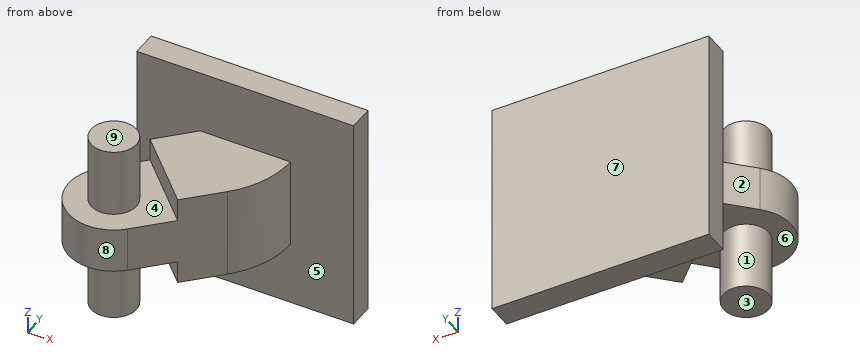
```python
from build123d import *

# Parameters (mm, degrees)
SKETCH_1_W           = 60
SKETCH_1_H           = 60
EXTRUDE_1_DEPTH      = 7
EXTRUDE_2_DEPTH      = 12.5
EXTRUDE_2_DEPTH_BACK = 12.5
CUT_EXTRUDE_START    = -12.5
CUT_EXTRUDE_1_DEPTH  = 6.25
CUT_EXTRUDE_START_2  = 6.25
CUT_EXTRUDE_2_DEPTH  = 6.25
EXTRUDE_3_DEPTH      = 25
EXTRUDE_3_DEPTH_BACK = 25
SKETCH_5_R           = 6.25


with BuildPart() as part:
    # 草图1 → 凸台-拉伸1 (new body)
    with BuildSketch(Plane(origin=(0, 0, 0), x_dir=(1, 0, 0), z_dir=(0, 1, 0))):
        Rectangle(SKETCH_1_W, SKETCH_1_H)
    extrude(amount=EXTRUDE_1_DEPTH)

    # 草图2 → 凸台-拉伸2 (add, two sides: drawn at the far end of the back side and taken through both)
    with BuildSketch(Plane.XY.offset(-EXTRUDE_2_DEPTH_BACK)):
        with BuildLine():
            Line((-12.5, 0), (12.5, 0))
            ThreePointArc((12.5, 0), (10.596988313, -9.567085809), (5.17766953, -17.67766953))
            Line((5.17766953, -17.67766953), (-12.5, -35.355339059))
            ThreePointArc((-12.5, -35.355339059), (-30.17766953, -35.355339059), (-30.17766953, -17.67766953))
            Line((-30.17766953, -17.67766953), (-12.5, 0))
        make_face()
    extrude(amount=EXTRUDE_2_DEPTH + EXTRUDE_2_DEPTH_BACK)

    # 草图3 → 切除-拉伸1 (cut)
    with BuildSketch(Plane.XY.offset(CUT_EXTRUDE_START)):
        with BuildLine():
            Line((-21.338834765, -8.838834765), (-3.661165235, -26.516504294))
            Line((-3.661165235, -26.516504294), (-12.5, -35.355339059))
            ThreePointArc((-12.5, -35.355339059), (-30.17766953, -35.355339059), (-30.17766953, -17.67766953))
            Line((-30.17766953, -17.67766953), (-21.338834765, -8.838834765))
        make_face()
    extrude(amount=CUT_EXTRUDE_1_DEPTH, mode=Mode.SUBTRACT)

    # 草图4 → 切除-拉伸2 (cut)
    with BuildSketch(Plane.XY.offset(CUT_EXTRUDE_START_2)):
        with BuildLine():
            Line((-3.661165235, -26.516504294), (-21.338834765, -8.838834765))
            Line((-21.338834765, -8.838834765), (-30.17766953, -17.67766953))
            ThreePointArc((-30.17766953, -17.67766953), (-30.17766953, -35.355339059), (-12.5, -35.355339059))
            Line((-12.5, -35.355339059), (-3.661165235, -26.516504294))
        make_face()
    extrude(amount=CUT_EXTRUDE_2_DEPTH, mode=Mode.SUBTRACT)

    # 草图5 → 凸台-拉伸3 (add, two sides: drawn at the far end of the back side and taken through both)
    with BuildSketch(Plane.XY.offset(-EXTRUDE_3_DEPTH_BACK)):
        with Locations((-21.338834765, -26.516504294)):
            Circle(SKETCH_5_R)
    extrude(amount=EXTRUDE_3_DEPTH + EXTRUDE_3_DEPTH_BACK)


solid = part.part
```
CAD build for the part. Positions are in the model's coordinates, mm. Face numbers are marked on the shaded views. A direction names the side the tool comes from. Coordinates: 2 decimals unless noted, no trailing zeros. Write each loop counter-clockwise with the first axis right and the second up, starting at its lowest first coordinate (ties: lowest second). Pieces come first, ordered by that corner, then holes. Notation, with made-up numbers: (66.25, 49.25) -> (125.25, 49.25) arc R28 cw to (125.25, 68.25) -> close; hole circle Ø3 at (-0.75, 78). An arc over 180 degrees is marked (long way). Return JSON: item names as keys, results as strings. Group by question number.
Q1. Which spindle directions (+Z, -Z, +X, -X, +Y, -Y) get a long thin tool onto all of the face, cutting with end or side? Do the marked faces 1, 2, 3, 4 and 5. Say none if no direction does.
Q2. Cut at D-D, the plane y = -23.5. Give the cut face in (x, z), then the cut area to 3 significant figures.
Q3. Cut at C-C, the plane z = 4. Give the cut face in (x, y), then the cut area to 3 significant figures.
Q4. Cut at B-B, the plane x = -19. Give the cut face in (y, z).
Q5. Pull direction Y, two halves, no side cores. Call the marked faces 6, 7, 8 and 9: released by +Y, released by -Y, zero draft, split by the parting line, or undercut.
Q6. Drill centre lines: line 1 (Y direction, x = 13.5, z = -9.5); line 2 (Z direction, x = -16.5, y = -35); line 3 (X direction, y = -26.5, z = -15). Where is each one in solid material? Low to high.
Q7. Flat gauge pins, fed straight in: pin 1 (5 mm diameter, centred on y = -8.5, z = 7.5, fed in from -X); pin 2 (13.5 mm diameter, centred on x = -9, y = -18.5, fed in from -Z); pin 3 (2 mm diameter, centred on y = 5, z = 5, fed in from -X). Where does each tip first touch, or does it go through?
Q8. Cut at A-A, the plane z = -10. Give the cut face in (x, y).
Returned:
{
 "1": {"face 1": "-Z", "face 2": "+Z, -Z, -X", "face 3": "-Z, +X, -X, -Y", "face 4": "+Z", "face 5": "none"},
 "2": {"outline": "(-33.47, -6.25) -> (-26.81, -6.25) -> (-26.81, -25) -> (-15.86, -25) -> (-15.86, -6.25) -> (-6.68, -6.25) -> (-6.68, -12.5) -> (-0.64, -12.5) -> (-0.64, 12.5) -> (-6.68, 12.5) -> (-6.68, 6.25) -> (-15.86, 6.25) -> (-15.86, 25) -> (-26.81, 25) -> (-26.81, 6.25) -> (-33.47, 6.25) -> close", "area": "896 mm2"},
 "3": {"outline": "(-30.18, -17.68) arc R12.5 ccw to (-12.5, -35.36) -> (5.18, -17.68) arc R25 ccw to (12.5, 0) -> (30, 0) -> (30, 7) -> (-30, 7) -> (-30, 0) -> (-12.5, 0) -> close", "area": "1,540 mm2"},
 "4": {"outline": "(-38.8, -6.25) -> (-32.31, -6.25) -> (-32.31, -25) -> (-20.72, -25) -> (-20.72, -6.25) -> (-11.18, -6.25) -> (-11.18, -12.5) -> (-6.5, -12.5) -> (-6.5, 12.5) -> (-11.18, 12.5) -> (-11.18, 6.25) -> (-20.72, 6.25) -> (-20.72, 25) -> (-32.31, 25) -> (-32.31, 6.25) -> (-38.8, 6.25) -> close; (0, -30) -> (7, -30) -> (7, 30) -> (0, 30) -> close"},
 "5": {"face 6": "undercut", "face 7": "released by +Y", "face 8": "split by the parting line", "face 9": "zero draft"},
 "6": {"line 1": "y = 0 to 7", "line 2": "z = -6.25 to 6.25", "line 3": "x = -27.59 to -15.09"},
 "7": {"pin 1": "stops at x = -23.17", "pin 2": "stops at z = -12.5", "pin 3": "stops at x = -30"},
 "8": {"outline": "(-30, 0) -> (-12.5, 0) -> (-21.34, -8.84) -> (-3.66, -26.52) -> (5.18, -17.68) arc R25 ccw to (12.5, 0) -> (30, 0) -> (30, 7) -> (-30, 7) -> close; circle Ø12.5 at (-21.34, -26.52)"}
}
